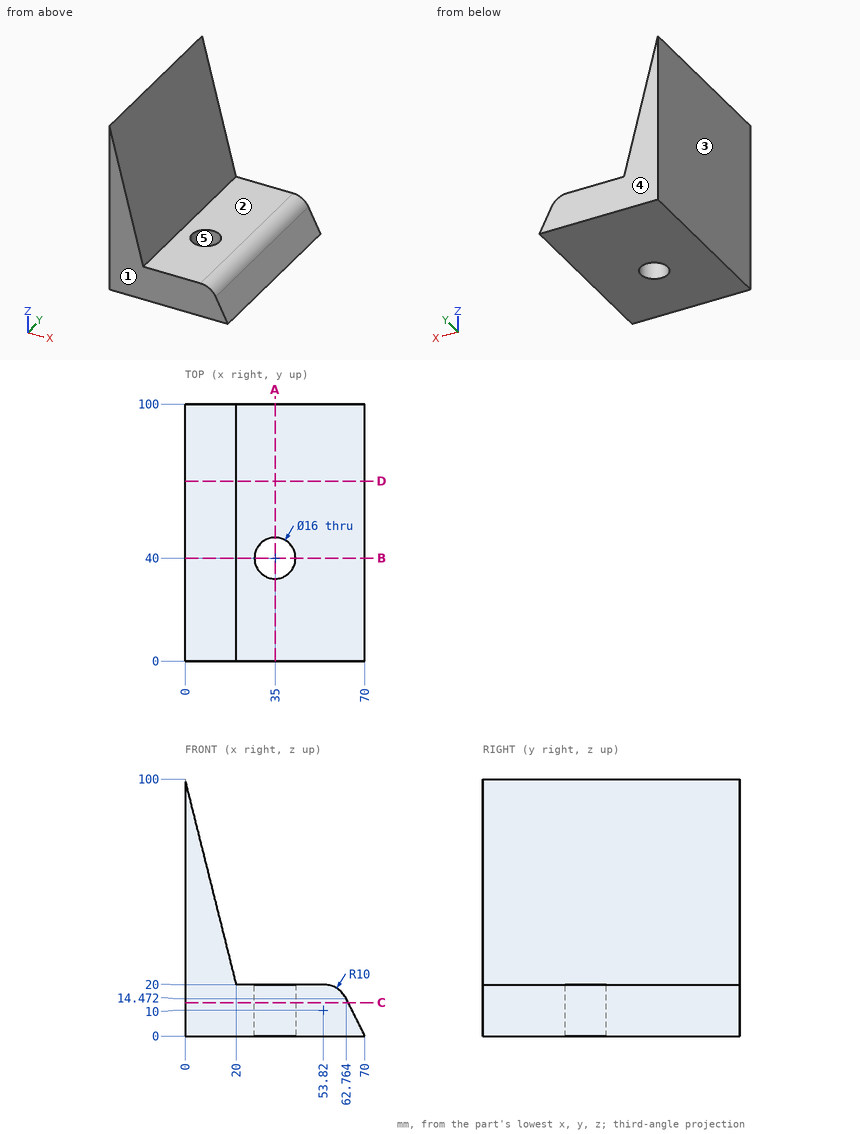
Print and shaded views of the part. All mm, measured from the part's lowest x, y and z. A direction names the side the tool comes from. Give positions to 0.01 mm unless a question says otherwise; leave off trailing zeros. Loops run counter-clockwise (first coordinate to the right, second up) from the corner with the lowest first, then second, coordinate; pieces in that order, holes last. Notation, with made-up numbers: (40.5, -13) -> (92.5, -13) arc R29 ccw to (92.5, 19) -> close; hole circle Ø1 at (65.5, 46). An arc over 180 degrees is marked (long way). One line per question, with ' | ' between items. Start each with the question number.
1) Cut at A-A (x = 35). Give the cut face in (y, z).
2) Two-plate mould, pull along Y, no slides. Class the marked faces 3, 4 and 5: released by +Y, released by -Y, zero draft, split by the parting line, or undercut.
3) 3-axis set-ups, long thin cutter, end or side, ignore diameter. For the marked faces 1 and 2: which of +Z, -Z, +X, -X, +Y, -Y reach the whole face in a straight line?
4) Cut at B-B (y = 40). Give the cut face in (x, z).
5) Cut at C-C (z = 13). Give the cut face in (x, y), plus the area to 3 significant figures.
6) Probe L1, parallel to Y at x = 35, z = 14; L2, parallel to Z at x = 43, y = 32; L3, parallel to X at y = 16.5, z = 23. List the from-to ranges inside material, lowest first.
7) Cut at D-D (y = 70). Give the cut face in (x, z).
Return value:
1) outline: (0, 0) -> (32, 0) -> (32, 20) -> (0, 20) -> close; (48, 0) -> (100, 0) -> (100, 20) -> (48, 20) -> close
2) face 3: zero draft | face 4: released by +Y | face 5: undercut
3) face 1: +Z, -Z, +X, -X, -Y | face 2: +Z, +X, +Y, -Y
4) outline: (0, 0) -> (27, 0) -> (27, 20) -> (20, 20) -> (0, 100) -> close; (43, 0) -> (70, 0) -> (62.76, 14.47) arc R10 ccw to (53.82, 20) -> (43, 20) -> close
5) outline: (0, 0) -> (63.5, 0) -> (63.5, 100) -> (0, 100) -> close; hole circle Ø16 at (35, 40) | area: 6,150 mm^2
6) L1: 0 to 32, 48 to 100 | L2: 0 to 20 | L3: 0 to 19.25
7) outline: (0, 0) -> (70, 0) -> (62.76, 14.47) arc R10 ccw to (53.82, 20) -> (20, 20) -> (0, 100) -> close
